The figure shows three views and two pictorial views of one solid part (mm, origin at its lowest corner). Answer the questions. A direction names the side the tool comes from. Give positions to 0.01 mm unless a question says otherwise; leave off trailing zeros. Write each loop counter-clockwise with the first axis right and the second up, starting at its lowest first coordinate (ties: lowest second). Pieces come first, ordered by that corner, then holes. Notation, with made-up numbers: (30, -15.5) -> (63, -15.5) arc R7 ccw to (63, -5.5) -> close; hole circle Ø5 at (59, 56). An arc over 180 degrees is marked (long way). Use a Markdown table: item, result.
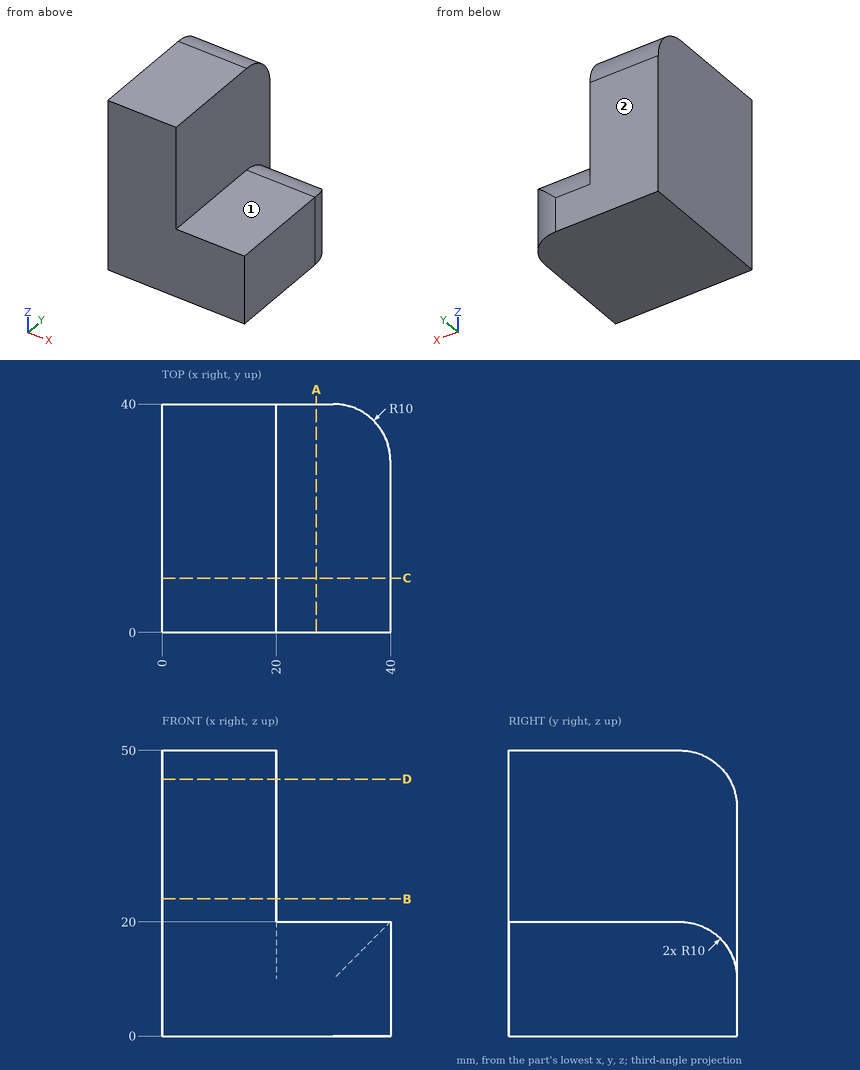
Item 1: A cutting plane is placed at C-C (y = 9.5). Give the vertices of the cut face in (x, z), then the cut area to 3 significant figures.
Return value:
| item | result |
|---|---|
| outline | (0, 0) -> (40, 0) -> (40, 20) -> (20, 20) -> (20, 50) -> (0, 50) -> close |
| area | 1,400 mm^2 |
Item 2: A cutting plane is placed at A-A (x = 27). Give the vertices of the cut face in (y, z).
Return value:
| item | result |
|---|---|
| outline | (0, 0) -> (40, 0) -> (40, 10) arc R10 ccw to (30, 20) -> (0, 20) -> close |
Item 3: A cutting plane is placed at D-D (z = 45). Give the vertices of the cut face in (x, y).
Return value:
| item | result |
|---|---|
| outline | (0, 0) -> (20, 0) -> (20, 38.66) -> (0, 38.66) -> close |
Item 4: A cutting plane is placed at B-B (z = 24). Give the vertices of the cut face in (x, y), then the cut area to 3 significant figures.
Return value:
| item | result |
|---|---|
| outline | (0, 0) -> (20, 0) -> (20, 40) -> (0, 40) -> close |
| area | 800 mm^2 |
Item 5: A tool of negligible diameter and unlimited length cuts with its end or side. For the marked faces 1 and 2, from which of +Z, -Z, +X, -X, +Y, -Y can it reach the whole face along a straight path? Write none if from no direction.
Return value:
| item | result |
|---|---|
| face 1 | +Z, +X, +Y, -Y |
| face 2 | +Z, -Z, +X, -X, +Y |
Item 6: Straight lines are drawn through the part: line 1 along X through (y, z) = (30, 25); line 2 along Y through (x, z) = (28, 10.5). For each, find the intervals that lie inside material, in ascending order. Write a range as [from, to].
Return value:
| item | result |
|---|---|
| line 1 | [0, 20] |
| line 2 | [0, 39.99] |
Item 7: Each of these flat-tipped pins is pushed along its axis until it touches: P1, Ø12, axis at y = 14, z = 43.5, coming from the +X side; P2, Ø2, axis at x = 34.5, y = 9, coming from the +Z side; P3, Ø2, axis at x = 10.5, y = 33, coming from the +Z side. Where does it stop, or does it pass through?
Return value:
| item | result |
|---|---|
| P1 | x = 20 |
| P2 | z = 20 |
| P3 | z = 49.8 |
